Here's the drawing with two shaded views (mm, measured from the low corner). I have some questions. Round coordinates to 2 decimals unless told otherwise and drop trailing zeros. Write each loop counter-clockwise with the first axis right and the second up, starting at its lowest first coordinate (ties: lowest second). Pieces come first, ordered by that corner, then holes. Notation, with made-up numbers: (11.5, 54) - (40.5, 54) arc R17 cw to (40.5, 68) - close; hole circle Ø4 at (-15.75, 82). An arc over 180 degrees is marked (long way). Return JSON: item names as keys, results as strings. Group by question number.
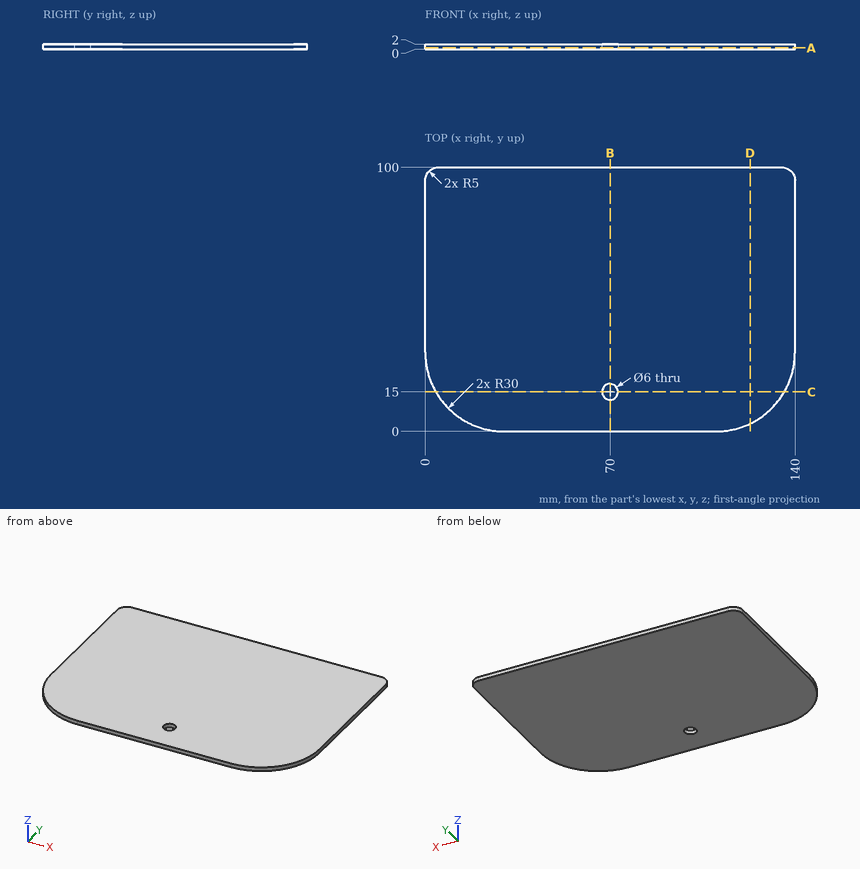
1) Imagine slicing it at A-A (z = 0.55). Please give me the cut outline in (x, y), plus the area to 3 significant figures.
2) I need wall thicknesses on line 1 along X through (y, z) = (29, 1.85); line 2 along Y through (x, z) = (127, 0.25); line 3 along Y through (x, z) = (68.5, 1.6). Which ranges of each line are inside material? Lowest first, please.
3) Imagine slicing it at C-C (y = 15). Please give me the cut outline in (x, z), plus the area to 3 significant figures.
4) Will these pins go through, and if not, where does the flat tip stop? pin 1 Ø1 at (y, z) = (28, 0.5) entering from +X; pin 2 Ø1 at (x, y) = (62, 67) entering from -Z.
5) Imagine slicing it at D-D (x = 123). Please give me the cut outline in (y, z), plus the area to 3 significant figures.
6) Imagine slicing it at B-B (x = 70). Please give me the cut outline in (y, z), plus the area to 3 significant figures.
Results found:
{
 "1": {"outline": "(0, 30) arc R30 ccw to (30, 0) - (110, 0) arc R30 ccw to (140, 30) - (140, 95) arc R5 ccw to (135, 100) - (5, 100) arc R5 ccw to (0, 95) - close; hole circle Ø6 at (70, 15)", "area": "13,600 mm²"},
 "2": {"line 1": "x = 0.02 to 139.98", "line 2": "y = 5.28 to 100", "line 3": "y = 0 to 12.4, 17.6 to 100"},
 "3": {"outline": "(4.02, 0) - (67, 0) - (67, 2) - (4.02, 2) - close; (73, 0) - (135.98, 0) - (135.98, 2) - (73, 2) - close", "area": "252 mm²"},
 "4": {"pin 1": "stops at x = 139.96", "pin 2": "stops at z = 0"},
 "5": {"outline": "(2.96, 0) - (100, 0) - (100, 2) - (2.96, 2) - close", "area": "194 mm²"},
 "6": {"outline": "(0, 0) - (12, 0) - (12, 2) - (0, 2) - close; (18, 0) - (100, 0) - (100, 2) - (18, 2) - close", "area": "188 mm²"}
}
